Input: part model. Units: mm. Frame: model coordinates. A direction names the side the tool comes from. Coordinates: 2 decimals unless noted, no trailing zeros. Loops run counter-clockwise (first coordinate to the right, second up) from the corner with the lowest first, then second, coordinate; pieces in that order, holes last.
```python
from build123d import *

# Parameters (mm, degrees)
SKETCH1_R           = 5.6945
SKETCH1_R_2         = 3.75
BOSS_EXTRUDE1_DEPTH = 5.2
BOSS_EXTRUDE3_START = -5.2
BOSS_EXTRUDE3_DEPTH = 5.2
FILLET1_R           = 1
FILLET2_R           = 1
CUT_EXTRUDE1_START  = -2
CUT_EXTRUDE1_DEPTH  = 2


with BuildPart() as part:
    # Sketch1 → Boss-Extrude1 (new body)
    with BuildSketch(Plane(origin=(0, 0, 0), x_dir=(1, 0, 0), z_dir=(0, 1, 0))):
        with Locations(Location((0, 0, 0), (0, 0, 270))):
            Circle(SKETCH1_R)
        with Locations(Location((0, 0, 0), (0, 0, 270))):
            Circle(SKETCH1_R_2, mode=Mode.SUBTRACT)
    extrude(amount=BOSS_EXTRUDE1_DEPTH)

    # Sketch2 → Boss-Extrude3 (add)
    with BuildSketch(Plane(origin=(0, 5.2, 0), x_dir=(1, 0, 0), z_dir=(0, 1, 0)).offset(BOSS_EXTRUDE3_START)):
        with BuildLine():
            Line((1.276851128, 5.549502811), (1.745257837, 7.585311288))
            add(Edge.make_bspline(
                [(1.745257837, 7.585311288), (1.554411596, 8.589760917), (1.089783036, 9.55790996), (0.435527939, 10.344585757)],
                knots=[0, 0, 0, 0, 1, 1, 1, 1], degree=3))
            ThreePointArc((0.435527939, 10.344585757), (0, 10.35375), (-0.435527939, 10.344585757))
            add(Edge.make_bspline(
                [(-1.745257837, 7.585311288), (-1.554411596, 8.589760917), (-1.089783036, 9.55790996), (-0.435527939, 10.344585757)],
                knots=[0, 0, 0, 0, 1, 1, 1, 1], degree=3))
            Line((-1.745257837, 7.585311288), (-1.276851128, 5.549502811))
            ThreePointArc((-1.276851128, 5.549502811), (0, 5.6945), (1.276851128, 5.549502811))
        make_face()
        with BuildLine():
            Line((3.021220978, 4.826961161), (4.129541397, 6.597708701))
            add(Edge.make_bspline(
                [(4.129541397, 6.597708701), (4.974743213, 7.173013173), (5.987869972, 7.529055922), (7.006761978, 7.622691496)],
                knots=[0, 0, 0, 0, 1, 1, 1, 1], degree=3))
            ThreePointArc((7.006761978, 7.622691496), (7.321206836, 7.321206836), (7.622691496, 7.006761978))
            add(Edge.make_bspline(
                [(6.597708701, 4.129541397), (7.173013173, 4.974743213), (7.529055922, 5.987869972), (7.622691496, 7.006761978)],
                knots=[0, 0, 0, 0, 1, 1, 1, 1], degree=3))
            Line((6.597708701, 4.129541397), (4.826961161, 3.021220978))
            ThreePointArc((4.826961161, 3.021220978), (4.026619565, 4.026619565), (3.021220978, 4.826961161))
        make_face()
        with BuildLine():
            Line((5.549502811, 1.276851128), (7.585311288, 1.745257837))
            add(Edge.make_bspline(
                [(7.585311288, 1.745257837), (8.589760917, 1.554411596), (9.55790996, 1.089783036), (10.344585757, 0.435527939)],
                knots=[0, 0, 0, 0, 1, 1, 1, 1], degree=3))
            ThreePointArc((10.344585757, 0.435527939), (10.35375, 0), (10.344585757, -0.435527939))
            add(Edge.make_bspline(
                [(7.585311288, -1.745257837), (8.589760917, -1.554411596), (9.55790996, -1.089783036), (10.344585757, -0.435527939)],
                knots=[0, 0, 0, 0, 1, 1, 1, 1], degree=3))
            Line((7.585311288, -1.745257837), (5.549502811, -1.276851128))
            ThreePointArc((5.549502811, -1.276851128), (5.6945, 0), (5.549502811, 1.276851128))
        make_face()
        with BuildLine():
            Line((4.826961161, -3.021220978), (6.597708701, -4.129541397))
            add(Edge.make_bspline(
                [(6.597708701, -4.129541397), (7.173013173, -4.974743213), (7.529055922, -5.987869972), (7.622691496, -7.006761978)],
                knots=[0, 0, 0, 0, 1, 1, 1, 1], degree=3))
            ThreePointArc((7.622691496, -7.006761978), (7.321206836, -7.321206836), (7.006761978, -7.622691496))
            add(Edge.make_bspline(
                [(4.129541397, -6.597708701), (4.974743213, -7.173013173), (5.987869972, -7.529055922), (7.006761978, -7.622691496)],
                knots=[0, 0, 0, 0, 1, 1, 1, 1], degree=3))
            Line((4.129541397, -6.597708701), (3.021220978, -4.826961161))
            ThreePointArc((3.021220978, -4.826961161), (4.026619565, -4.026619565), (4.826961161, -3.021220978))
        make_face()
        with BuildLine():
            Line((1.276851128, -5.549502811), (1.745257837, -7.585311288))
            add(Edge.make_bspline(
                [(1.745257837, -7.585311288), (1.554411596, -8.589760917), (1.089783036, -9.55790996), (0.435527939, -10.344585757)],
                knots=[0, 0, 0, 0, 1, 1, 1, 1], degree=3))
            ThreePointArc((0.435527939, -10.344585757), (0, -10.35375), (-0.435527939, -10.344585757))
            add(Edge.make_bspline(
                [(-1.745257837, -7.585311288), (-1.554411596, -8.589760917), (-1.089783036, -9.55790996), (-0.435527939, -10.344585757)],
                knots=[0, 0, 0, 0, 1, 1, 1, 1], degree=3))
            Line((-1.745257837, -7.585311288), (-1.276851128, -5.549502811))
            ThreePointArc((-1.276851128, -5.549502811), (0, -5.6945), (1.276851128, -5.549502811))
        make_face()
        with BuildLine():
            Line((-3.021220978, -4.826961161), (-4.129541397, -6.597708701))
            add(Edge.make_bspline(
                [(-4.129541397, -6.597708701), (-4.974743213, -7.173013173), (-5.987869972, -7.529055922), (-7.006761978, -7.622691496)],
                knots=[0, 0, 0, 0, 1, 1, 1, 1], degree=3))
            ThreePointArc((-7.006761978, -7.622691496), (-7.321206836, -7.321206836), (-7.622691496, -7.006761978))
            add(Edge.make_bspline(
                [(-6.597708701, -4.129541397), (-7.173013173, -4.974743213), (-7.529055922, -5.987869972), (-7.622691496, -7.006761978)],
                knots=[0, 0, 0, 0, 1, 1, 1, 1], degree=3))
            Line((-6.597708701, -4.129541397), (-4.826961161, -3.021220978))
            ThreePointArc((-4.826961161, -3.021220978), (-4.026619565, -4.026619565), (-3.021220978, -4.826961161))
        make_face()
        with BuildLine():
            Line((-5.549502811, -1.276851128), (-7.585311288, -1.745257837))
            add(Edge.make_bspline(
                [(-7.585311288, -1.745257837), (-8.589760917, -1.554411596), (-9.55790996, -1.089783036), (-10.344585757, -0.435527939)],
                knots=[0, 0, 0, 0, 1, 1, 1, 1], degree=3))
            ThreePointArc((-10.344585757, -0.435527939), (-10.35375, 0), (-10.344585757, 0.435527939))
            add(Edge.make_bspline(
                [(-7.585311288, 1.745257837), (-8.589760917, 1.554411596), (-9.55790996, 1.089783036), (-10.344585757, 0.435527939)],
                knots=[0, 0, 0, 0, 1, 1, 1, 1], degree=3))
            Line((-7.585311288, 1.745257837), (-5.549502811, 1.276851128))
            ThreePointArc((-5.549502811, 1.276851128), (-5.6945, 0), (-5.549502811, -1.276851128))
        make_face()
        with BuildLine():
            Line((-4.826961161, 3.021220978), (-6.597708701, 4.129541397))
            add(Edge.make_bspline(
                [(-6.597708701, 4.129541397), (-7.173013173, 4.974743213), (-7.529055922, 5.987869972), (-7.622691496, 7.006761978)],
                knots=[0, 0, 0, 0, 1, 1, 1, 1], degree=3))
            ThreePointArc((-7.622691496, 7.006761978), (-7.321206836, 7.321206836), (-7.006761978, 7.622691496))
            add(Edge.make_bspline(
                [(-4.129541397, 6.597708701), (-4.974743213, 7.173013173), (-5.987869972, 7.529055922), (-7.006761978, 7.622691496)],
                knots=[0, 0, 0, 0, 1, 1, 1, 1], degree=3))
            Line((-4.129541397, 6.597708701), (-3.021220978, 4.826961161))
            ThreePointArc((-3.021220978, 4.826961161), (-4.026619565, 4.026619565), (-4.826961161, 3.021220978))
        make_face()
    extrude(amount=BOSS_EXTRUDE3_DEPTH)

    # Fillet1
    fillet1_edges = [part.edges().sort_by_distance(p)[0] for p in [
        (1.276851128, 2.6, -5.549502811),
        (-1.276851128, 2.6, -5.549502811),
    ]]
    fillet(fillet1_edges, radius=FILLET1_R)

    # Fillet2
    fillet2_edges = [part.edges().sort_by_distance(p)[0] for p in [
        (-5.549502811, 2.6, -1.276851128),
        (-5.549502811, 2.6, 1.276851128),
        (-3.021220978, 2.6, -4.826961161),
        (-4.826961161, 2.6, -3.021220978),
        (4.826961161, 2.6, -3.021220978),
        (3.021220978, 2.6, -4.826961161),
        (5.549502811, 2.6, 1.276851128),
        (5.549502811, 2.6, -1.276851128),
        (3.021220978, 2.6, 4.826961161),
        (4.826961161, 2.6, 3.021220978),
        (-1.276851128, 2.6, 5.549502811),
        (1.276851128, 2.6, 5.549502811),
        (-4.826961161, 2.6, 3.021220978),
        (-3.021220978, 2.6, 4.826961161),
    ]]
    fillet(fillet2_edges, radius=FILLET2_R)

    # Sketch3 → Cut-Extrude1 (cut)
    with BuildSketch(Plane(origin=(0, 5.2, 0), x_dir=(1, 0, 0), z_dir=(0, 1, 0)).offset(CUT_EXTRUDE1_START)):
        with BuildLine():
            Line((0.356514085, 3.73301456), (14.428169014, 2.389129319))
            ThreePointArc((14.428169014, 2.389129319), (11.8, 0), (14.428169014, -2.389129319))
            Line((14.428169014, -2.389129319), (0.356514085, -3.73301456))
            ThreePointArc((0.356514085, -3.73301456), (3.75, 0), (0.356514085, 3.73301456))
        make_face()
    extrude(amount=CUT_EXTRUDE1_DEPTH, mode=Mode.SUBTRACT)


solid = part.part
```
Item 1: Section query A-A (z = 0). Output: boundary loops of the cut face in (x, y).
Result:
outline: (-10.35, 0) - (-3.75, 0) - (-3.75, 5.2) - (-10.35, 5.2) - close; (3.75, 0) - (10.35, 0) - (10.35, 3.2) - (3.75, 3.2) - close
Item 2: Contact query for flat-ended pins moving along their axis: P1, Ø2, axis at x = -7.5, y = 2, coming from the -Z side; P2, Ø3, axis at y = 1, z = -6.5, coming from the -X side; P3, Ø12, axis at x = 0, z = 0, coming from the -Y side; P4, Ø2, axis at x = 7, z = 0, coming from the +Y side. Output: stop coordinate, or through.
Result:
P1: stops at z = -7.62
P2: stops at x = -7.62
P3: stops at y = 0
P4: stops at y = 3.2
Item 3: Mould query, pull axis Z, two halves, no side actions, for faces 1 (the face through (1.613, 2.564, -7.01)), 2 (the face through (3.825, 2.564, 6.111)). Classes: +Z half, -Z half, draft (parallel to the pull), parting line (faces both ways), or undercut.
Result:
face 1: undercut
face 2: +Z half
Item 4: Section query C-C (x = 3). Output: boundary loops of the cut face in (y, z).
Result:
outline: (0, -5.2) - (5.2, -5.2) - (5.2, -3.48) - (3.2, -3.48) - (3.2, -2.25) - (0, -2.25) - close; (0, 2.25) - (3.2, 2.25) - (3.2, 3.48) - (5.2, 3.48) - (5.2, 5.2) - (0, 5.2) - close
Item 5: Reachability of faces 3 (the face through (-7.026, 2.564, -1.617)), 4 (the face through (3, 2.6, 5.2)), 5 (the face through (-6.111, 2.564, 3.825)), 6 (the face through (6.1, 2.56, 3.82)), 7 (the face through (5, 3.2, 0)) from +Z, -Z, +X, -X, +Y, -Y: full face, straight path, thin tool, end or side. Return the list, or none.
Result:
face 3: +Y, -Y
face 4: +Z, +Y, -Y
face 5: -X, +Y, -Y
face 6: +X, +Y, -Y
face 7: +Y
Item 6: Section query D-D (z = 6). Count the separate pieces of the cut face and the enclosed holes in it, then the cut area to 3 significant figures.
Result:
separate pieces: 3
enclosed holes: 0
area: 53.8 mm2
Item 7: Section query B-B (x = 0). Output: boundary loops of the cut face in (y, z).
Result:
outline: (0, -10.35) - (5.2, -10.35) - (5.2, -3.75) - (0, -3.75) - close; (0, 3.75) - (5.2, 3.75) - (5.2, 10.35) - (0, 10.35) - close
Item 8: Line query: L1, parallel to X at y = 2.6, z = 0; L2, parallel to Z at x = -5.25, y = 2.1. Output: solid intervals per line, ascending.
Result:
L1: x = -10.35 to -3.75, 3.75 to 10.35
L2: z = -7.19 to -3.12, -2.21 to 2.21, 3.12 to 7.19
